Autodesk Inventor part; units mm, degrees
ref_plane "YZ Plane" through (0, 0, 0) normal (1, 0, 0) x (0, 1, 0)
ref_plane "XZ Plane" through (0, 0, 0) normal (0, 1, 0) x (-1, 0, 0)
ref_plane "XY Plane" through (0, 0, 0) normal (0, 0, 1) x (1, 0, 0)
sketch "Sketch1" plane through (0, 0, 0) normal (0, 0, 1) x (1, 0, 0)
  arc A0 (-8.2061, -3.1475) -> (-7.8618, -4.0207) centre (-7.8531, -3.5128) ccw
  line L0 (-0.8184, 3.9914) -> (-8.2061, -3.1475)
  arc A1 (-0.4592, 4.1402) -> (-0.8184, 3.9914) centre (-0.4592, 3.6322) ccw
  line L1 (0.4145, 4.1402) -> (-0.4592, 4.1402)
  arc A2 (0.8488, 3.962) -> (0.4145, 4.1402) centre (0.4606, 3.6343) ccw
  line L2 (8.2061, -3.1475) -> (0.8488, 3.962)
  arc A3 (7.8618, -4.0207) -> (8.2061, -3.1475) centre (7.8531, -3.5128) ccw
  line L3 (-7.8618, -4.0207) -> (7.8618, -4.0207)
  circle A4 centre (21.4376, -2.3876) radius 2.032
  circle A5 centre (-21.4376, -2.3876) radius 2.032
  arc A6 (16.9463, 6.35) -> (15.8972, 5.301) centre (16.9463, 5.301) ccw
  line L4 (15.8972, 5.301) -> (15.8972, 5.1892)
  arc A7 (15.8972, 5.1892) -> (16.9463, 4.1402) centre (16.9463, 5.1892) ccw
  line L5 (16.9463, 4.1402) -> (19.0952, 4.1402)
  arc A8 (19.8159, 2.3571) -> (19.0952, 4.1402) centre (19.0952, 3.103) ccw
  line L6 (19.8159, 2.3571) -> (16.5346, -0.8136)
  arc A9 (14.3374, -1.7018) -> (16.5346, -0.8136) centre (14.3374, 1.4602) ccw
  line L7 (14.3374, -1.7018) -> (11.0626, -1.7018)
  arc A10 (8.8654, -0.8136) -> (11.0626, -1.7018) centre (11.0626, 1.4602) ccw
  line L8 (8.8654, -0.8136) -> (5.5841, 2.3571)
  arc A11 (6.3048, 4.1402) -> (5.5841, 2.3571) centre (6.3048, 3.103) ccw
  line L9 (6.3048, 4.1402) -> (8.4349, 4.1402)
  arc A12 (8.4349, 4.1402) -> (9.4839, 5.1892) centre (8.4349, 5.1892) ccw
  line L10 (9.4839, 5.1892) -> (9.4839, 5.301)
  arc A13 (9.4839, 5.301) -> (8.4349, 6.35) centre (8.4349, 5.301) ccw
  line L11 (8.4349, 6.35) -> (7.3479, 6.35)
  arc A14 (6.332, 6.35) -> (7.3479, 6.35) centre (6.8399, 6.3541) ccw
  line L12 (6.332, 6.35) -> (3.1719, 6.35)
  arc A15 (2.156, 6.35) -> (3.1719, 6.35) centre (2.6639, 6.3541) ccw
  line L13 (2.156, 6.35) -> (-2.156, 6.35)
  arc A16 (-3.1719, 6.35) -> (-2.156, 6.35) centre (-2.6639, 6.3541) ccw
  line L14 (-3.1719, 6.35) -> (-6.3893, 6.35)
  arc A17 (-7.4052, 6.35) -> (-6.3893, 6.35) centre (-6.8973, 6.3541) ccw
  line L15 (-7.4052, 6.35) -> (-8.4349, 6.35)
  arc A18 (-8.4349, 6.35) -> (-9.4839, 5.301) centre (-8.4349, 5.301) ccw
  line L16 (-9.4839, 5.301) -> (-9.4839, 5.1892)
  arc A19 (-9.4839, 5.1892) -> (-8.4349, 4.1402) centre (-8.4349, 5.1892) ccw
  line L17 (-8.4349, 4.1402) -> (-6.3048, 4.1402)
  arc A20 (-5.5841, 2.3571) -> (-6.3048, 4.1402) centre (-6.3048, 3.103) ccw
  line L18 (-5.5841, 2.3571) -> (-8.8654, -0.8136)
  arc A21 (-11.0626, -1.7018) -> (-8.8654, -0.8136) centre (-11.0626, 1.4602) ccw
  line L19 (-11.0626, -1.7018) -> (-14.3374, -1.7018)
  arc A22 (-16.5346, -0.8136) -> (-14.3374, -1.7018) centre (-14.3374, 1.4602) ccw
  line L20 (-16.5346, -0.8136) -> (-19.809, 2.3504)
  arc A23 (-19.0855, 4.1402) -> (-19.809, 2.3504) centre (-19.0855, 3.0991) ccw
  line L21 (-19.0855, 4.1402) -> (-17.0099, 4.1402)
  arc A24 (-17.0099, 4.1402) -> (-15.9609, 5.1892) centre (-17.0099, 5.1892) ccw
  line L22 (-15.9609, 5.1892) -> (-15.9609, 5.301)
  arc A25 (-15.9609, 5.301) -> (-17.0099, 6.35) centre (-17.0099, 5.301) ccw
  line L23 (-17.0099, 6.35) -> (-18.0395, 6.35)
  arc A26 (-19.0555, 6.35) -> (-18.0395, 6.35) centre (-18.5475, 6.3541) ccw
  line L24 (-19.0555, 6.35) -> (-22.2504, 6.35)
  arc A27 (-23.2664, 6.354) -> (-22.2504, 6.35) centre (-22.7584, 6.3541) ccw
  arc A28 (-23.2664, 6.354) -> (-25.4, 4.2459) centre (-23.2918, 4.2459) ccw
  line L25 (-25.4, 4.2459) -> (-25.4, -4.2459)
  arc A29 (-25.4, -4.2459) -> (-23.2881, -6.4371) centre (-23.2933, -4.3288) ccw
  arc A30 (-22.2765, -6.35) -> (-23.2881, -6.4371) centre (-22.7808, -6.4114) ccw
  line L26 (-22.2765, -6.35) -> (-19.0448, -6.35)
  arc A31 (-18.0363, -6.35) -> (-19.0448, -6.35) centre (-18.5406, -6.4114) ccw
  line L27 (-18.0363, -6.35) -> (-7.4084, -6.35)
  arc A32 (-6.3999, -6.35) -> (-7.4084, -6.35) centre (-6.9041, -6.4114) ccw
  line L28 (-6.3999, -6.35) -> (-3.1684, -6.35)
  arc A33 (-2.1599, -6.35) -> (-3.1684, -6.35) centre (-2.6641, -6.4114) ccw
  line L29 (-2.1599, -6.35) -> (2.1135, -6.35)
  arc A34 (3.122, -6.35) -> (2.1135, -6.35) centre (2.6177, -6.4114) ccw
  line L30 (3.122, -6.35) -> (6.3882, -6.35)
  arc A35 (7.3967, -6.35) -> (6.3882, -6.35) centre (6.8925, -6.4114) ccw
  line L31 (7.3967, -6.35) -> (18.0231, -6.35)
  arc A36 (19.0317, -6.35) -> (18.0231, -6.35) centre (18.5274, -6.4114) ccw
  line L32 (19.0317, -6.35) -> (22.2866, -6.35)
  arc A37 (23.2982, -6.4371) -> (22.2866, -6.35) centre (22.7909, -6.4114) ccw
  arc A38 (23.2982, -6.4371) -> (25.4, -4.2459) centre (23.2933, -4.3288) ccw
  line L33 (25.4, -4.2459) -> (25.4, 4.2355)
  arc A39 (25.4, 4.2355) -> (23.2665, 6.354) centre (23.2918, 4.2459) ccw
  arc A40 (22.2505, 6.35) -> (23.2665, 6.354) centre (22.7585, 6.3541) ccw
  line L34 (22.2505, 6.35) -> (18.998, 6.35)
  arc A41 (17.9823, 6.35) -> (18.998, 6.35) centre (18.4902, 6.3374) ccw
  line L35 (17.9823, 6.35) -> (16.9463, 6.35)
  point P0 (0, 0)
extrude "Extrusion1" add sketch "Sketch1" against normal blind 304.8
properties part number "2012-BLACK-FB"
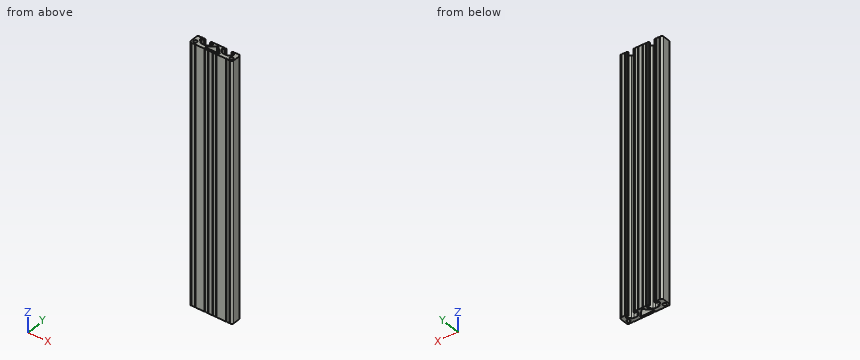
CAD build for the part. Positions are in the model's coordinates, mm. Round coordinates to 2 decimals unless told otherwise and drop trailing zeros. Write item = value, one per line. Start each with the question number.
Q1. Band-saw the part on A-A (z = -112). Count the separate pieces of the cut face and the enclosed holes in it, then the cut area to 3 significant figures.
Q2. Drop flat-ended pins along their axis: pin 1 (0.8 mm diameter, centred on x = -17.5, z = -202.5, fed in from +Y); pin 2 (5.5 mm diameter, centred on x = -11.5, z = -136.5, fed in from -Y). Give the stop position or say it passes through.
Q3. Probe L1, parallel to Y at x = 0, z = -170; L2, parallel to Y at x = 16.5, z = -72.5; L3, parallel to X at y = 0.75, z = -118. List the from-to ranges inside material, lowest first. Write a range as from..to.
Answers below:
q1.separate_pieces = 1
q1.enclosed_holes = 3
q1.area = 368 mm2
q2.pin_1 = 6.35
q2.pin_2 = -6.35
q3.L1 = -6.35..-4.02, 4.14..6.35
q3.L2 = -6.35..-0.85, 4.24..6.25
q3.L3 = -25.4..-18.15, -7.25..-4.17, 4.17..7.25, 18.15..25.4
